Job drawing, mm, ordinate dimensions from the low corner. One solid piece. A direction names the side the tool comes from. Coordinates: 2 decimals unless noted, no trailing zeros. Loops run counter-clockwise (first coordinate to the right, second up) from the corner with the lowest first, then second, coordinate; pieces in that order, holes last. Notation, with made-up numbers: (68, 19) - (76, 19) arc R19 ccw to (76, 24) - close; hole circle Ø2 at (-6, 24.5). An arc over 180 degrees is marked (long way). One line per question, with ' | ' between items. Start each with the question number.
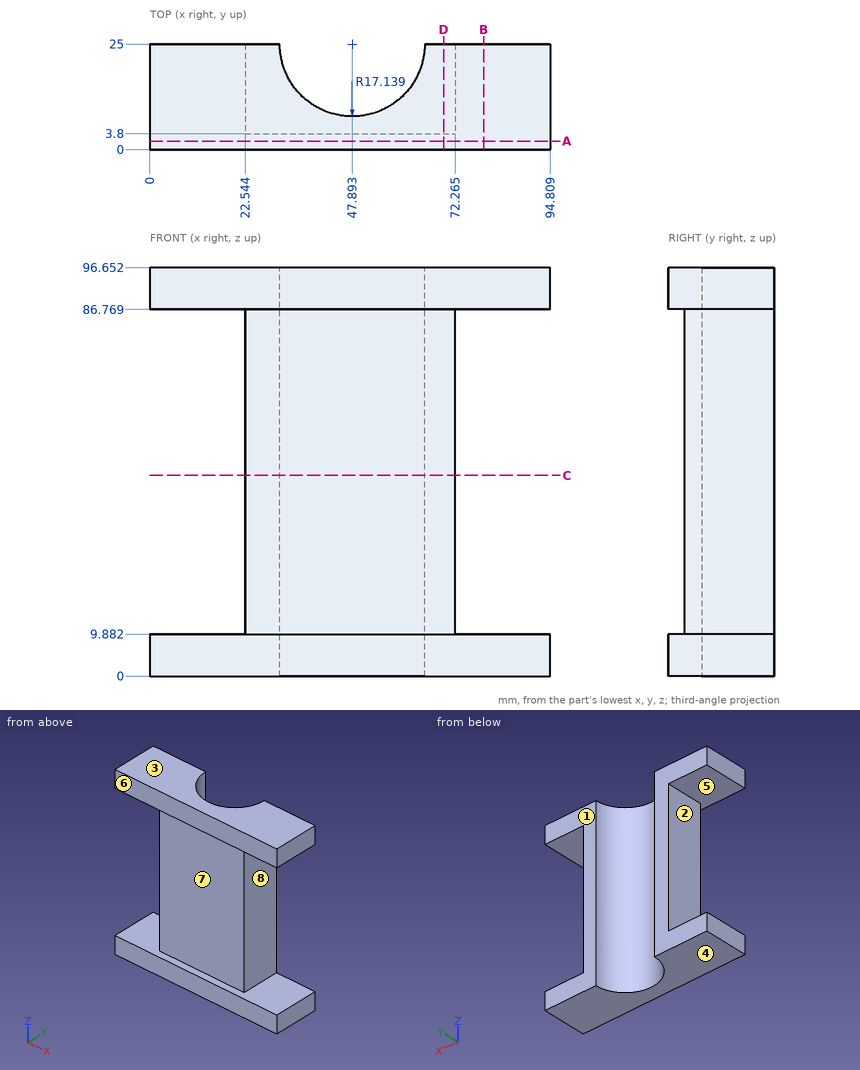
1) Band-saw the part on D-D on x = 69.5. List the corners of the cut face in (y, z), then the cut area to 3 significant figures.
2) Band-saw the part on A-A on y = 2. List the corners of the cut face in (x, z), then the cut area to 3 significant figures.
3) Tool access for the marked faces 5, 6, 7 and 8: list every direction of +Z, -Z, +X, -X, +Y, -Y with a clear straight run to the whole face (end or side of a thin tool).
4) Mould opens along Z. For the marked faces 1, 2, 3 and 4 say: +Z half, -Z half, draft (parallel to the pull), parting line (faces both ways), or undercut.
5) Wall check: line 1 along Z through (x, y) = (85.5, 8); line 2 along X through (y, z) = (21, 64.5) (1 decimal); line 3 along X through (y, z) = (7.25, 17) (1 decimal). Give the ranges that are in metal, low to high. Write a range as [from, to].
6) Band-saw the part on B-B on x = 79. List the corners of the cut face in (y, z).
7) Band-saw the part on C-C on z = 47.5. List the corners of the cut face in (x, y) (1 decimal), then the cut area to 3 significant figures.
8) Pin check, flat tips, straight feed: pin 1 Ø4 at (x, y) = (64.5, 9) entering from -Z; pin 2 Ø4 at (y, z) = (11.5, 44) entering from -X; pin 3 Ø6 at (x, z) = (44, 23) entering from -Y. Stop position of each tip, or through.
Values found:
1) outline: (0, 0) - (25, 0) - (25, 96.65) - (0, 96.65) - (0, 86.77) - (3.8, 86.77) - (3.8, 9.88) - (0, 9.88) - close | area: 2,120 mm²
2) outline: (0, 0) - (94.81, 0) - (94.81, 9.88) - (0, 9.88) - close; (0, 86.77) - (94.81, 86.77) - (94.81, 96.65) - (0, 96.65) - close | area: 1,870 mm²
3) face 5: -Y | face 6: +Z, -Z, +X, -X, -Y | face 7: +X, -X, -Y | face 8: +X, +Y, -Y
4) face 1: draft | face 2: undercut | face 3: +Z half | face 4: -Z half
5) line 1: [0, 9.88], [86.77, 96.65] | line 2: [22.5, 31.2], [64.6, 72.3] | line 3: [22.5, 72.3]
6) outline: (0, 0) - (25, 0) - (25, 9.88) - (0, 9.88) - close; (0, 86.77) - (25, 86.77) - (25, 96.65) - (0, 96.65) - close
7) outline: (22.5, 3.8) - (72.3, 3.8) - (72.3, 25) - (65, 25) arc R17.1 cw to (30.8, 25) - (22.5, 25) - close | area: 593 mm²
8) pin 1: z = 0 | pin 2: x = 22.54 | pin 3: y = 3.8
